Input: part model. Units: mm. Frame: model coordinates. A direction names the side the tool comes from. Give positions to 0.01 mm unless a question says otherwise; leave off trailing zeros. Loops run counter-clockwise (first coordinate to the right, second up) from the corner with the lowest first, then second, coordinate; pieces in that order, holes last. Notation, with made-up numbers: (-35.5, 70.5) -> (-0.5, 70.5) arc R20 ccw to (-0.5, 93.5) -> close; hole circle Ø9 at (42.5, 40.25). An arc over 180 degrees is marked (long way). Answer as a JSON object with one key per item and string values. Group by question number.
```python
from build123d import *

# Parameters (mm, degrees)
SKETCH1_R           = 150
BOSS_EXTRUDE1_DEPTH = 75
CHAMFER1_SIZE       = 10
SKETCH2_W           = 70
SKETCH2_H           = 70
BOSS_EXTRUDE2_DEPTH = 10
CHAMFER2_SIZE       = 10


with BuildPart() as part:
    # Sketch1 → Boss-Extrude1 (new body)
    with BuildSketch(Plane(origin=(0, 0, 0), x_dir=(1, 0, 0), z_dir=(0, 1, 0))):
        Circle(SKETCH1_R)
    extrude(amount=BOSS_EXTRUDE1_DEPTH)

    # Chamfer1
    chamfer1_edges = [part.edges().sort_by_distance(p)[0] for p in [
        (-150, 75, 0),
    ]]
    chamfer(chamfer1_edges, length=CHAMFER1_SIZE)

    # Sketch2 → Boss-Extrude2 (add)
    with BuildSketch(Plane.XZ):
        with Locations((-150, 0)):
            Rectangle(SKETCH2_W, SKETCH2_H)
    extrude(amount=-BOSS_EXTRUDE2_DEPTH)

    # Chamfer2
    chamfer2_edges = [part.edges().sort_by_distance(p)[0] for p in [
        (-185, 5, 35),
    ]]
    chamfer(chamfer2_edges, length=CHAMFER2_SIZE)


solid = part.part
```
Q1. Section C-C on x = -154. Return the cut outline in (y, z).
Q2. Ray query, probe 1 along X at (y, z) = (29, 5); probe 2 along Z at (x, y) = (68, 41.5); probe 3 along Z at (x, y) = (-12.5, 55). Return the intervals inside material, ascending.
Q3. Section A-A on z = 0. Return the cut outline in (x, y), then the cut area to 4 significant figures.
Q4. Section B-B on y = 51. Return the cut outline in (x, z).
Q5. Set-up query: faces 1 (the face through (-161, 5, 35)), 2 (the face through (-166, 5, -35)), 3 (the face through (-2, 75, -2)). Return all of +Z, -Z, +X, -X, +Y, -Y with unobstructed straight access to the full face (end or side cutting, diameter ignored); none if empty.
Q6. Pin query (flat end, axial travel): pin 1 Ø1.5 at (y, z) = (55, -20.5) entering from +X; pin 2 Ø6 at (x, y) = (33.5, 12) entering from -Z; pin 3 Ø1 at (y, z) = (11, 21.5) entering from +X. Return the tip coordinate at first contact, or that it passes through.
Numbers:
{
 "1": {"outline": "(0, -35) -> (10, -35) -> (10, 35) -> (0, 35) -> close"},
 "2": {"probe 1": "x = -149.92 to 149.92", "probe 2": "z = -133.7 to 133.7", "probe 3": "z = -149.48 to 149.48"},
 "3": {"outline": "(-185, 0) -> (150, 0) -> (150, 65) -> (140, 75) -> (-140, 75) -> (-150, 65) -> (-150, 10) -> (-185, 10) -> close", "area": "22,750 mm²"},
 "4": {"outline": "circle Ø300 at (0, 0)"},
 "5": {"face 1": "+Z, -X, +Y, -Y", "face 2": "-Z, -X, +Y, -Y", "face 3": "+Z, -Z, +X, -X, +Y"},
 "6": {"pin 1": "stops at x = 148.69", "pin 2": "stops at z = -146.87", "pin 3": "stops at x = 148.52"}
}
